The listing builds one solid part. Answer for the finished solid, in the listing's coordinates (mm). A direction names the side the tool comes from. Give positions to 0.01 mm unless a question says otherwise; leave off trailing zeros. Order: outer loops, then holes, each group sorted by start corner. A loop starts at its lowest first (then second) coordinate and runs counter-clockwise, first axis right, second up. Notation, with made-up numbers: (2, 22.5) -> (50, 22.5) arc R20 cw to (50, 31.5) -> close; hole circle Ø3 at (47, 56.5). An arc over 180 degrees is marked (long way). One line per question, with ' | ' between items. Start each with the question number.
```python
from build123d import *

# Parameters (mm, degrees)
SKETCH1_R                = 8
BOSS_EXTRUDE1_DEPTH      = 10
BOSS_EXTRUDE2_DEPTH      = 1
BOSS_EXTRUDE2_DEPTH_BACK = 41
SKETCH2_R                = 25
SKETCH2_R_2              = 14
BOSS_EXTRUDE3_DEPTH      = 16


with BuildPart() as part:
    # Sketch1 → Boss-Extrude1 (new body)
    with BuildSketch(Plane(origin=(0, 0, 0), x_dir=(1, 0, 0), z_dir=(0, 1, 0))):
        with BuildLine():
            Line((0, 30.616062134), (-71, 30.616062134))
            Line((-71, 30.616062134), (-71, -30.616062134))
            ThreePointArc((-71, -30.616062134), (-62.398661132, -49.486247959), (-42.513286954, -55.371724761))
            Line((-42.513286954, -55.371724761), (49.486713046, -42.413978282))
            ThreePointArc((49.486713046, -42.413978282), (64.870185825, -34.056976787), (71, -17.658315655))
            Line((71, -17.658315655), (71, 30.616062134))
            Line((71, 30.616062134), (0, 30.616062134))
        make_face()
        with Locations(Location((46, -9.383937866, 0), (0, 0, 270))):
            Circle(SKETCH1_R, mode=Mode.SUBTRACT)
        with Locations(Location((-46, -34.383937866, 0), (0, 0, 270))):
            Circle(SKETCH1_R, mode=Mode.SUBTRACT)
    extrude(amount=BOSS_EXTRUDE1_DEPTH)



with BuildPart() as body_2:
    # Sketch2 → Boss-Extrude2 (new, two sides: drawn at the far end of the back side and taken through both)
    with BuildSketch(Plane.XY.offset(-BOSS_EXTRUDE2_DEPTH_BACK)):
        with Locations((-46, 75)):
            Circle(SKETCH2_R)
        with Locations((-46, 75)):
            Circle(SKETCH2_R_2, mode=Mode.SUBTRACT)
    extrude(amount=BOSS_EXTRUDE2_DEPTH + BOSS_EXTRUDE2_DEPTH_BACK)


with BuildPart() as part_1:
    add(part.part)

    add(body_2.part)  # Boss-Extrude3 merges body 2
    # Sketch3 → Boss-Extrude3 (add)
    with BuildSketch(Plane(origin=(0, 0, -30.616062134), x_dir=(-1, 0, 0), z_dir=(0, 0, -1))):
        with BuildLine():
            Line((21, 10), (71, 10))
            Line((71, 10), (71, 75))
            ThreePointArc((71, 75), (46, 50), (21, 75))
            Line((21, 75), (21, 10))
        make_face()
    extrude(amount=-BOSS_EXTRUDE3_DEPTH)


solid = part_1.part
```
(1) The part is cut by section C-C on z = -22.5. Determine the outline of the cut face in (x, y), plus the area to 3 significant figures.
(2) Determine the mould class of faces 6 (the face through (-1, 10, 12)), 7 (the face through (-40.59, 4.93, 28.49)), 8 (the face through (64.7, 4.93, 34.25)) for opening direction Z: pulls with the +Z half, pulls with the -Z half, needs draft (parallel to the pull), parting line crosses it, or undercut.
(3) For faces 1 (the face through (-47.82, 88.88, -20.29)), 2 (the face through (-21, 43, -23)), 3 (the face through (2.843, 4.93, 48.984)), 4 (the face through (-49.255, 99.787, -20.294)), 5 (the face through (-35, 64, 1)), determine the directions among +Z, -Z, +X, -X, +Y, -Y from which every point of the face is accessible in a straight line to the end or side of a thin tool.
(4) Consider line 1 (Y direction, x = -57, z = -2); line 2 (X direction, y = 76, z = -32); line 3 (X direction, y = 16, z = -21). Determine where each line is inside the solid, lowest interval first.
(5) The part is cut by section B-B on z = -7. Determine the outline of the cut face in (x, y).
(6) Given P1, Ø25, axis at x = -58, y = 82, coming from the +Z side; P2, Ø6, axis at x = -32.5, y = 25, coming from the +Z side; P3, Ø21, axis at x = -46, z = 34.38, coming from the +Y side; P4, Ø14.5, axis at x = 46, z = 9.38, coming from the +Y side (3 decimals), each flat-ended and moving along its own axis, determine where each tip first touches the part or whether it passes through.
(7) The part is cut by section D-D on x = 46. Determine the outline of the cut face in (y, z).
(8) The part is cut by section A-A on x = -46. Determine the outline of the cut face in (y, z), plus the area to 3 significant figures.
Result sheet:
1) outline: (-71, 0) -> (71, 0) -> (71, 10) -> (-21, 10) -> (-21, 75) arc R25 ccw to (-71, 75) -> close; hole circle Ø28 at (-46, 75) | area: 5,040 mm^2
2) face 6: needs draft | face 7: undercut | face 8: pulls with the +Z half
3) face 1: +Z, -Z | face 2: +Z, -Z, +X, +Y | face 3: +Z, +X, +Y, -Y | face 4: none | face 5: +Z, +X, -X, +Y
4) line 1: y = 0 to 10, 52.55 to 66.34, 83.66 to 97.45 | line 2: x = -70.98 to -59.96, -32.04 to -21.02 | line 3: x = -71 to -21
5) outline: (-71, 0) -> (71, 0) -> (71, 10) -> (-71, 10) -> close; circle Ø50 at (-46, 75); hole circle Ø28 at (-46, 75)
6) P1: stops at z = 1 | P2: stops at z = -14.62 | P3: stops at y = 10 | P4: passes through
7) outline: (0, -30.62) -> (10, -30.62) -> (10, 1.38) -> (0, 1.38) -> close; (0, 17.38) -> (10, 17.38) -> (10, 42.91) -> (0, 42.91) -> close
8) outline: (0, -30.62) -> (50, -30.62) -> (50, -41) -> (61, -41) -> (61, 1) -> (50, 1) -> (50, -14.62) -> (10, -14.62) -> (10, 26.38) -> (0, 26.38) -> close; (0, 42.38) -> (10, 42.38) -> (10, 55.62) -> (0, 55.62) -> close; (89, -41) -> (100, -41) -> (100, 1) -> (89, 1) -> close | area: 2,270 mm^2
